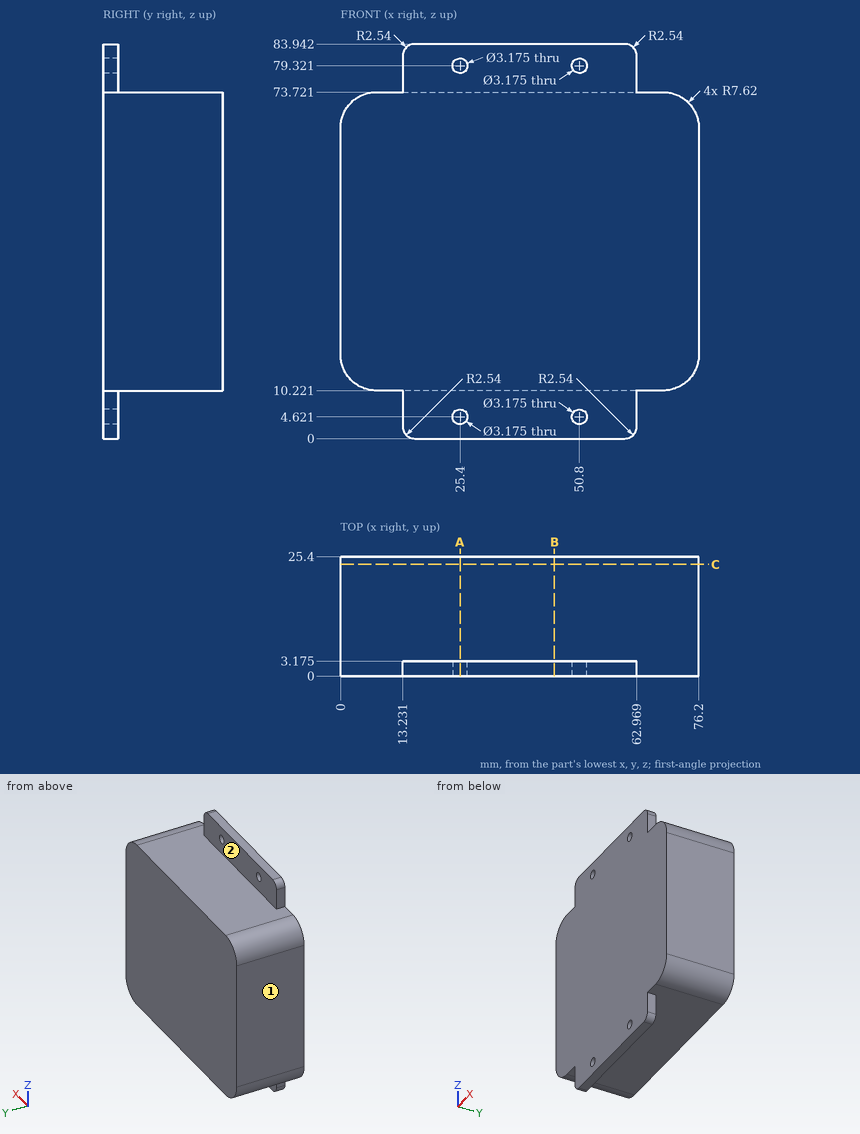
Study the drawing (mm; zero at the part's minimum x, y, z) and answer. A direction names the side the tool comes from. Give positions to 0.01 mm unless a question says otherwise; leave off trailing zeros. Order: outer loops, then holes, each group sorted by start corner. A loop starts at its lowest first (then second) coordinate and runs counter-clockwise, first axis right, second up.
1. For the marked faces 1 and 2, determine the directions among +Z, -Z, +X, -X, +Y, -Y from which every point of the face is accessible in a straight line to the end or side of a thin tool.
Result sheet:
face 1: +Z, -Z, -X, +Y, -Y
face 2: +Z, +X, -X, +Y
2. Section C-C, the plane y = 23.75 is taken. Determine the outline of the cut face in (x, z).
Result sheet:
outline: (0, 17.84) arc R7.62 ccw to (7.62, 10.22) - (68.58, 10.22) arc R7.62 ccw to (76.2, 17.84) - (76.2, 66.1) arc R7.62 ccw to (68.58, 73.72) - (7.62, 73.72) arc R7.62 ccw to (0, 66.1) - close
3. Section B-B, the plane x = 45.5 is taken. Determine the outline of the cut face in (y, z) (1 decimal), and give its area (3 significant figures).
Result sheet:
outline: (0, 0) - (3.2, 0) - (3.2, 10.2) - (25.4, 10.2) - (25.4, 73.7) - (3.2, 73.7) - (3.2, 83.9) - (0, 83.9) - close
area: 1,680 mm2
4. Section A-A, the plane x = 25.4 is taken. Determine the outline of the cut face in (y, z) (1 decimal), and give its area (3 significant figures).
Result sheet:
outline: (0, 0) - (3.2, 0) - (3.2, 3) - (0, 3) - close; (0, 6.2) - (3.2, 6.2) - (3.2, 10.2) - (25.4, 10.2) - (25.4, 73.7) - (3.2, 73.7) - (3.2, 77.7) - (0, 77.7) - close; (0, 80.9) - (3.2, 80.9) - (3.2, 83.9) - (0, 83.9) - close
area: 1,660 mm2
5. Each of these flat-tipped pins is pushed along its axis until it touches: P1, Ø8, axis at x = 19, y = 21, coming from the +Z side; P2, Ø2.5, axis at y = 1, z = 6, coming from the -X side; P3, Ø10, axis at y = 6, z = 11.5, coming from the -X side; P4, Ø4, axis at x = 29, z = 23.5, coming from the -Y side. Where does it stop, or does it pass through?
Result sheet:
P1: stops at z = 73.72
P2: stops at x = 13.23
P3: stops at x = 0.12
P4: stops at y = 0
6. Straight lines are drawn through the part: L1, parallel to Z at x = 50.8, y = 1.2; L2, parallel to X at y = 2.75, z = 80.5 (1 decimal); L3, parallel to Z at x = 42, y = 16.25. For each, find the intervals that lie inside material, in ascending order.
Result sheet:
L1: z = 0 to 3.03, 6.21 to 77.73, 80.91 to 83.94
L2: x = 13.2 to 24.3, 26.5 to 49.7, 51.9 to 63
L3: z = 10.22 to 73.72
